Here's how the part is built. I have some questions about the finished solid (model axes, mm). A direction names the side the tool comes from. Give positions to 0.01 mm unless a question says otherwise; leave off trailing zeros. Write each loop counter-clockwise with the first axis right and the second up, starting at its lowest first coordinate (ties: lowest second). Pieces come first, ordered by that corner, then holes. Notation, with made-up numbers: M 75,-27 L 107,-27 A15 cw 107,-9 Z; hole C -35.5,-34 d4. An arc over 180 degrees is marked long. Answer as CSV lines item,"result". Start each with the question number.
Q1. Thinking about a two-plate mould opening in X: for faces 3 (the flat face through (-11, -17.5, 1)), 4 (the flat face through (5.5, -15, 1)), 5 (the cylindrical face through (-18.9, 11.93, 0.81)), 6 (the flat face through (19.5, -2, 1)), which applies, +X half, -X half, draft (parallel to the pull), parting line (faces both ways), or undercut?
Q2. Suppose I cut it at C-C (x = -1.5). Write out the boundary of the cut face in (y, z), then the cut area to 3 significant figures.
Q3. If I drill on line 1 along X through (y, z) = (-12.75, 0.4); line 2 along Y through (x, z) = (-2.5, 1.2), over which ranges is the centre line in solid material (lowest first)?
Q4. On a 3-axis mill with a long thin cutter (end or side, diameter ignored), from which of +Z, -Z, +X, -X, +Y, -Y can I reach the whole of each face in a straight line? I mean faces 1 (the flat face through (0, -12.5, 1)), 2 (the cylindrical face through (18.9, -16.93, 0.81)). Say none if no direction works.
Q5. Suppose I cut it at B-B (z = 0.75). Write out the boundary of the cut face in (x, y), then the cut area to 3 significant figures.
Q6. Suppose I cut it at A-A (y = -13.25). Write out the boundary of the cut face in (x, z).
Autodesk Inventor part; units mm, degrees
ref_plane "YZ Plane" through (0, 0, 0) normal (1, 0, 0) x (0, 1, 0)
ref_plane "XZ Plane" through (0, 0, 0) normal (0, 1, 0) x (-1, 0, 0)
ref_plane "XY Plane" through (0, 0, 0) normal (0, 0, 1) x (1, 0, 0)
sketch "Sketch2" plane through (0, 0, 0) normal (0, 0, 1) x (1, 0, 0)
  line L0 (-19.4999, -12.4999) -> (-19.4999, 12.4999)
  line L1 (-19.4999, 12.4999) -> (19.4999, 12.4999)
  line L2 (19.4999, 12.4999) -> (19.4999, -12.4999)
  line L3 (19.4999, -12.4999) -> (-19.4999, 12.4999) construction
  line L4 (-19.4999, -12.4999) -> (19.4999, 12.4999) construction
  line L5 (-5.4999, -12.4999) -> (-5.4999, -17.4996)
  line L6 (-5.4999, -17.4996) -> (-19.4999, -17.4996)
  line L7 (-19.4999, -17.4996) -> (-19.4999, -12.4999)
  line L8 (5.4995, -12.4999) -> (5.4995, -17.4996)
  line L9 (5.4995, -17.4996) -> (19.4999, -17.4996)
  line L10 (19.4999, -17.4996) -> (19.4999, -12.4999)
  line L11 (-5.4999, -12.4999) -> (5.4995, -12.4999)
  point P0 (0, 0)
extrude "Extrusion2" add sketch "Sketch2" along normal blind 1.6
fillet "Fillet3" radius 2 4 edges at (19.4999, 12.4999, 0.8) (-19.4999, 12.4999, 0.8) (19.4999, -17.4996, 0.8) (-19.4999, -17.4996, 0.8)
properties part number "pcb_balun_top"
Resolved:
1,face 3,"draft"
1,face 4,"undercut"
1,face 5,"-X half"
1,face 6,"+X half"
2,outline,"M -12.5,0 L 12.5,0 L 12.5,1.6 L -12.5,1.6 Z"
2,area,"40.0 mm^2"
3,line 1,"-19.5 to -5.5, 5.5 to 19.5"
3,line 2,"-12.5 to 12.5"
4,face 1,"+Z, -Z, -Y"
4,face 2,"+Z, -Z, +X, -Y"
5,outline,"M -19.5,-15.5 A2 ccw -17.5,-17.5 L -5.5,-17.5 L -5.5,-12.5 L 5.5,-12.5 L 5.5,-17.5 L 17.5,-17.5 A2 ccw 19.5,-15.5 L 19.5,10.5 A2 ccw 17.5,12.5 L -17.5,12.5 A2 ccw -19.5,10.5 Z"
5,area,"1,110 mm^2"
6,outline,"M -19.5,0 L -5.5,0 L -5.5,1.6 L -19.5,1.6 Z; M 5.5,0 L 19.5,0 L 19.5,1.6 L 5.5,1.6 Z"
